Source: CAD feature listing. Evaluate the final solid. Frame: model axes, mm. A direction names the side the tool comes from. Coordinates: 2 decimals unless noted, no trailing zeros. Order: outer loops, then holes, each group sorted by start corner. A loop starts at its lowest first (then second) coordinate and runs counter-clockwise, first axis right, second up.
Autodesk Fusion 360 part; units mm, degrees
sketch "Sketch1" plane through (0, 0, 0) normal (0, 0, 1) x (1, 0, 0)
  circle A0 centre (0, 0) radius 15.24
  circle A1 centre (0, 0) radius 20.32
  line L0 (18.6388, 8.093) -> (57.15, 8.093)
  line L1 (57.15, 8.093) -> (57.15, -9.687)
  line L2 (57.15, -9.687) -> (17.8624, -9.687)
  line L3 (0, 15.24) -> (0, -15.24) construction
  line L4 (-18.6388, 8.093) -> (-57.15, 8.093)
  line L5 (-57.15, 8.093) -> (-57.15, -9.687)
  line L6 (-57.15, -9.687) -> (-17.8624, -9.687)
  circle A2 centre (-47.1067, 0) radius 3.81
  circle A3 centre (47.1067, 0) radius 3.81
  dimension "d1" = 30.48
  dimension "d2" = 5.08
  dimension "d3" = 57.15
  dimension "d4" = 17.78
  dimension "d11" = 7.62
extrude "Extrude1" add sketch "Sketch1" along normal blind 15.24 contours A0 | A1
extrude "Extrude2" add sketch "Sketch1" along normal blind 3.81 contours A1 L0 L1 L2 | A1 L4 L5 L6 | A2 | A3
fillet "Fillet1" radius 5.08 4 edges at (57.15, 8.093, 1.905) (57.15, -9.687, 1.905) (-57.15, 8.093, 1.905) (-57.15, -9.687, 1.905)
extrude "Extrude3" cut sketch "Sketch1" along normal blind 5.08 contours A2 | A3
extrude "Extrude4" cut sketch "Sketch1" along normal blind 10.16 contours A0
fillet "Fillet2" radius 2.54 1 edges at (-18.9449, -7.348, 15.24)
Q1. Set-up query: faces 1 (the flat face through (0, 0, 10.16)), 2 (the flat face through (35, 8.093, 2)), 3 (the cylindrical face through (-20.3, -0.9, 6.3)), 4 (the flat face through (35, -9.687, 2)), 5 (the flat face through (-35, 8.093, 2)). Return all of +Z, -Z, +X, -X, +Y, -Y with unobstructed straight access to the full face (end or side cutting, diameter ignored); none if empty.
Solutions:
face 1: -Z
face 2: +Z, -Z, +X, +Y
face 3: +Z
face 4: +Z, -Z, +X, -Y
face 5: +Z, -Z, -X, +Y
Q2. Section query B-B on x = 0. Output: boundary loops of the cut face in (y, z), plus the area to 3 significant figures.
Solutions:
outline: (-20.32, 0) - (-15.24, 0) - (-15.24, 10.16) - (15.24, 10.16) - (15.24, 0) - (20.32, 0) - (20.32, 12.7) arc R2.54 ccw to (17.78, 15.24) - (-17.78, 15.24) arc R2.54 ccw to (-20.32, 12.7) - close
area: 307 mm2
Q3. Section query C-C on z = 8.75. Output: boundary loops of the cut face in (x, y).
Solutions:
outline: circle Ø40.64 at (0, 0); hole circle Ø30.48 at (0, 0)
Q4. Section query A-A on y = 0. Output: boundary loops of the cut face in (x, z), plus the area to 3 significant figures.
Solutions:
outline: (-57.15, 0) - (-50.92, 0) - (-50.92, 3.81) - (-57.15, 3.81) - close; (-43.3, 0) - (-15.24, 0) - (-15.24, 10.16) - (15.24, 10.16) - (15.24, 0) - (43.3, 0) - (43.3, 3.81) - (20.32, 3.81) - (20.32, 12.7) arc R2.54 ccw to (17.78, 15.24) - (-17.78, 15.24) arc R2.54 ccw to (-20.32, 12.7) - (-20.32, 3.81) - (-43.3, 3.81) - close; (50.92, 0) - (57.15, 0) - (57.15, 3.81) - (50.92, 3.81) - close
area: 529 mm2
Q5. Section query D-D on x = -40.5. Output: boundary loops of the cut face in (y, z), plus the area to 3 significant figures.
Solutions:
outline: (-9.69, 0) - (8.09, 0) - (8.09, 3.81) - (-9.69, 3.81) - close
area: 67.7 mm2
Q6. Material intervals for line 1 along Y through (x, z) = (0, 8); line 2 along Z through (x, y) = (7, -9); line 3 along Y through (x, z) = (12, 3), sorted ascending.
Solutions:
line 1: y = -20.32 to -15.24, 15.24 to 20.32
line 2: z = 10.16 to 15.24
line 3: y = -16.4 to -9.39, 9.39 to 16.4
Q7. Pull-direction query (Y, two-part tool) for faces 6 (the cylindrical face through (43.3, -0.2, 1.9)), 7 (the flat face through (-35, -9.687, 2)), 8 (the flat face through (-38, -1, 3.81)), 9 (the cylindrical face through (-3.3, 14.88, 5.01)); classes: pulls with the +Y half, pulls with the -Y half, needs draft (parallel to the pull), parting line crosses it, or undercut.
Solutions:
face 6: undercut
face 7: pulls with the -Y half
face 8: needs draft
face 9: undercut
Q8. Pin query (flat end, axial travel): P1, Ø9, axis at x = -47.11, y = 0, coming from the +Z side; P2, Ø1.5, axis at y = 9, z = 9, coming from the -X side; P3, Ø4, axis at x = 41, z = 1.5, coming from the -Y side. Return the tip coordinate at first contact, or that it passes through.
Solutions:
P1: stops at z = 3.81
P2: stops at x = -18.57
P3: stops at y = -9.69
